Can you work these out from the model? Positions are in its coordinate system, mm. A direction names the side the tool comes from. Round coordinates to 2 decimals unless told otherwise and drop trailing zeros. Order: outer loops, then holes, each group sorted by start corner. A loop starts at its lowest first (then second) coordinate and runs counter-clockwise, first axis right, second up. Notation, with made-up numbers: M 6.25,41.25 L 27.25,41.25 A6 cw 27.25,48.25 Z; hole C -4,78.5 d5. An arc over 180 degrees is marked long. One line per question, with ' | ' between items.
```python
from build123d import *

# Parameters (mm, degrees)
BOSS_EXTRUDE1_DEPTH = 50
SKETCH2_R           = 52
BOSS_EXTRUDE2_DEPTH = 67
SKETCH3_R           = 43
BOSS_EXTRUDE3_DEPTH = 3
CUT_EXTRUDE1_REACH  = 322
SKETCH4_R           = 24
SKETCH5_R           = 33
CUT_EXTRUDE2_DEPTH  = 4
BOSS_EXTRUDE4_DEPTH = 248
SKETCH7_R           = 3
CUT_EXTRUDE3_DEPTH  = 248
BOSS_EXTRUDE5_DEPTH = 20
SKETCH9_R           = 50
BOSS_EXTRUDE6_DEPTH = 20
CUT_EXTRUDE4_REACH  = 22
FILLET1_R           = 25
CUT_EXTRUDE5_DEPTH  = 34
SKETCH12_W          = 78
SKETCH12_H          = 64
CUT_EXTRUDE6_DEPTH  = 240
SKETCH13_W          = 12
SKETCH13_H          = 110
CUT_EXTRUDE7_DEPTH  = 240


with BuildPart() as part:
    # Sketch1 → Boss-Extrude1 (new body, symmetric)
    with BuildSketch(Plane(origin=(0, 0, 0), x_dir=(0, 0, -1), z_dir=(1, 0, 0))):
        with BuildLine():
            Line((-226, 0), (54, 0))
            Line((54, 0), (54, 20))
            Line((54, 20), (52, 20))
            Line((52, 20), (52, 80))
            Line((52, 80), (20, 80))
            Line((20, 80), (20, 74))
            Line((20, 74), (-20, 74))
            Line((-20, 74), (-20, 80))
            Line((-20, 80), (-58, 80))
            Line((-58, 80), (-58, 250))
            Line((-58, 250), (0, 250))
            Line((0, 250), (0, 317))
            Line((0, 317), (-58, 317))
            ThreePointArc((-58, 317), (-114.640297133, 296.941952651), (-146.034066228, 245.708372014))
            Line((-146.034066228, 245.708372014), (-194, 20))
            Line((-194, 20), (-226, 20))
            Line((-226, 20), (-226, 0))
        make_face()
    extrude(amount=BOSS_EXTRUDE1_DEPTH, both=True)

    # Sketch2 → Boss-Extrude2 (add)
    with BuildSketch(Plane(origin=(0, 317, 0), x_dir=(1, 0, 0), z_dir=(0, 1, 0))):
        Circle(SKETCH2_R)
    extrude(amount=-BOSS_EXTRUDE2_DEPTH)

    # Sketch3 → Boss-Extrude3 (add)
    with BuildSketch(Plane(origin=(0, 317, 0), x_dir=(1, 0, 0), z_dir=(0, 1, 0))):
        Circle(SKETCH3_R)
    extrude(amount=BOSS_EXTRUDE3_DEPTH)

    # Sketch4 → Cut-Extrude1 (cut, up to next)
    with BuildSketch(Plane(origin=(0, 320, 0), x_dir=(1, 0, 0), z_dir=(0, 1, 0)), mode=Mode.PRIVATE) as cut_extrude1_sk1:
        Circle(SKETCH4_R)
    cut_extrude1_tool1 = extrude(cut_extrude1_sk1.sketch, amount=-CUT_EXTRUDE1_REACH, mode=Mode.PRIVATE) & part.part
    add(cut_extrude1_tool1.solids().sort_by_distance((0, 320, 0))[0], mode=Mode.SUBTRACT)

    # Sketch5 → Cut-Extrude2 (cut)
    with BuildSketch(Plane.XZ.offset(-250)):
        Circle(SKETCH5_R)
    extrude(amount=-CUT_EXTRUDE2_DEPTH, mode=Mode.SUBTRACT)

    # Sketch6 → Boss-Extrude4 (add, symmetric)
    with BuildSketch(Plane(origin=(0, 0, 0), x_dir=(0, 0, -1), z_dir=(1, 0, 0))):
        Polygon((-58, 80), (-58, 0), (54, 0), (54, 20), (52, 20), (52, 80), (20, 80), (20, 74), (-20, 74), (-20, 80), align=None)
    extrude(amount=BOSS_EXTRUDE4_DEPTH, both=True)

    # Sketch7 → Cut-Extrude3 (cut, symmetric)
    with BuildSketch(Plane(origin=(0, 0, 0), x_dir=(0, 0, -1), z_dir=(1, 0, 0))):
        with Locations((-55, 80)):
            Circle(SKETCH7_R)
    extrude(amount=CUT_EXTRUDE3_DEPTH, both=True, mode=Mode.SUBTRACT)

    # Sketch8 → Boss-Extrude5 (add)
    with BuildSketch(Plane.XZ):
        with BuildLine():
            Line((-272, 12.5), (-303.006817759, 12.5))
            ThreePointArc((-303.006817759, 12.5), (-192, 2), (-303.006817759, -8.5))
            Line((-303.006817759, -8.5), (-272, -8.5))
            ThreePointArc((-272, -8.5), (-261.5, 2), (-272, 12.5))
        make_face()
        with BuildLine():
            Line((272, -8.5), (303.006817759, -8.5))
            ThreePointArc((303.006817759, -8.5), (192, 2), (303.006817759, 12.5))
            Line((303.006817759, 12.5), (272, 12.5))
            ThreePointArc((272, 12.5), (261.5, 2), (272, -8.5))
        make_face()
    extrude(amount=-BOSS_EXTRUDE5_DEPTH)

    # Sketch9 → Boss-Extrude6 (add)
    with BuildSketch(Plane(origin=(0, 20, 0), x_dir=(1, 0, 0), z_dir=(0, 1, 0))):
        with Locations((0, -226)):
            Circle(SKETCH9_R)
    extrude(amount=-BOSS_EXTRUDE6_DEPTH)

    # Sketch10 → Cut-Extrude4 (cut, up to next)
    with BuildSketch(Plane(origin=(0, 20, 0), x_dir=(1, 0, 0), z_dir=(0, 1, 0)), mode=Mode.PRIVATE) as cut_extrude4_sk1:
        with BuildLine():
            ThreePointArc((10.5, -226), (0, -215.5), (-10.5, -226))
            Line((-10.5, -226), (-10.5, -291))
            ThreePointArc((-10.5, -291), (0, -301.5), (10.5, -291))
            Line((10.5, -291), (10.5, -226))
        make_face()
    cut_extrude4_tool1 = extrude(cut_extrude4_sk1.sketch, amount=-CUT_EXTRUDE4_REACH, mode=Mode.PRIVATE) & part.part
    add(cut_extrude4_tool1.solids().sort_by_distance((0, 20, 258.5))[0], mode=Mode.SUBTRACT)

    # Fillet1
    fillet1_edges = [part.edges().sort_by_distance(p)[0] for p in [
        (0, 250, 58),
    ]]
    fillet(fillet1_edges, radius=FILLET1_R)

    # Sketch11 → Cut-Extrude5 (cut, symmetric)
    with BuildSketch(Plane(origin=(0, 0, 0), x_dir=(0, 0, -1), z_dir=(1, 0, 0))):
        with BuildLine():
            Line((-130.383565565, 242.382439212), (-181.892953201, 0))
            Line((-181.892953201, 0), (0, 0))
            Line((0, 0), (0, 64))
            Line((0, 64), (-74, 64))
            Line((-74, 64), (-74, 225))
            ThreePointArc((-74, 225), (-61.991378029, 253.991378029), (-33, 266))
            Line((-33, 266), (-33, 301))
            Line((-33, 301), (-58, 301))
            ThreePointArc((-58, 301), (-104.570910976, 284.507827735), (-130.383565565, 242.382439212))
        make_face()
    extrude(amount=CUT_EXTRUDE5_DEPTH, both=True, mode=Mode.SUBTRACT)

    # Sketch12 → Cut-Extrude6 (cut, symmetric)
    with BuildSketch(Plane(origin=(0, 0, 0), x_dir=(0, 0, -1), z_dir=(1, 0, 0))):
        with Locations((-3, 32)):
            Rectangle(SKETCH12_W, SKETCH12_H)
    extrude(amount=CUT_EXTRUDE6_DEPTH, both=True, mode=Mode.SUBTRACT)

    # Sketch13 → Cut-Extrude7 (cut, symmetric)
    with BuildSketch(Plane(origin=(0, 0, 58), x_dir=(-1, 0, 0), z_dir=(0, 0, -1))):
        with Locations((14, 170)):
            Rectangle(SKETCH13_W, SKETCH13_H)
        with Locations((-14, 170)):
            Rectangle(SKETCH13_W, SKETCH13_H)
    extrude(amount=CUT_EXTRUDE7_DEPTH, both=True, mode=Mode.SUBTRACT)


solid = part.part
```
(1) If we section it at C-C on y = 199: Please give me the cut outline in (x, z), plus the area to 3 significant figures.
Final values:
outline: M -50,58 L -20,58 L -20,74 L -34,74 L -34,139.6 L -20,139.6 L -20,155.96 L -50,155.96 Z; M -8,58 L 8,58 L 8,74 L -8,74 Z; M -8,139.6 L 8,139.6 L 8,155.96 L -8,155.96 Z; M 20,58 L 50,58 L 50,155.96 L 20,155.96 L 20,139.6 L 34,139.6 L 34,74 L 20,74 Z | area: 4,560 mm^2
(2) Thinking about a two-plate mould opening in Y: for faces 5 (the flat face through (14, 225, 142)), 6 (the flat face through (8, 169, 66)), 7 (the flat face through (-14, 115, 166)), 8 (the flat face through (-20, 169, 154)), which applies, released by +Y, released by -Y, zero draft, split by the parting line, or undercut?
Final values:
face 5: released by -Y | face 6: undercut | face 7: released by +Y | face 8: zero draft
(3) If we section it at B-B on z = 0: Please give me the cut outline in (x, y), plus the area to 3 significant figures.
Final values:
outline: M -261.69,0 L -240,0 L -240,64 L 240,64 L 240,0 L 261.69,0 L 261.69,20 L 248,20 L 248,74 L -248,74 L -248,20 L -261.69,20 Z; M -52,250 L -33,250 L -33,254 L -24,254 L -24,320 L -43,320 L -43,317 L -52,317 Z; M 24,254 L 33,254 L 33,250 L 52,250 L 52,317 L 43,317 L 43,320 L 24,320 Z | area: 10,300 mm^2
(4) On a 3-axis mill with a long thin cutter (end or side, diameter ignored), from which of +Z, -Z, +X, -X, +Y, -Y can I reach the whole of each face in a straight line? I mean faces 1 (the flat face through (-14, 115, 66)), 2 (the cylindrical face through (0.48, 253.67, 62.31)), 3 (the cylindrical face through (-5.598, 318.479, -42.634)), 4 (the flat face through (-14, 225, 142)). Say none if no direction works.
Final values:
face 1: +Z, -Z | face 2: none | face 3: +Y | face 4: +Z, -Z, -Y
(5) Will these pins go through, and if not, where does the flat tip stop? pin 1 Ø22 at (x, y) = (-282, 12) entering from -Z; pin 2 Ø9.5 at (x, z) = (-15, 69.5) entering from +Y; pin 3 Ø12 at (y, z) = (45, 75) entering from +X.
Final values:
pin 1: z = -49.06 | pin 2: y = 316.75 | pin 3: x = 50
(6) If we section it at D-D on x = -227.5: Please give me the cut outline in (y, z), plus the area to 3 significant figures.
Final values:
outline: M 0,-54 L 20,-54 L 20,-52 L 80,-52 L 80,-20 L 74,-20 L 74,20 L 80,20 L 80,52 A3 cw 80,58 L 0,58 L 0,42 L 64,42 L 64,-36 L 0,-36 Z | area: 3,590 mm^2
(7) If we section it at A-A on z = 246: Please give me the cut outline in (x, y).
Final values:
outline: M -45.83,0 L -10.5,0 L -10.5,20 L -45.83,20 Z; M 10.5,0 L 45.83,0 L 45.83,20 L 10.5,20 Z
(8) Please list where these lines run through material, in increasing order: probe 1 along Z at (x, y) = (-69, 59); probe 2 along X at (y, z) = (14, 112); probe 3 along X at (y, z) = (283, 0). Write a range as [from, to].
Final values:
probe 1: [-52, -36], [42, 58] | probe 2: [-50, -34], [34, 50] | probe 3: [-52, -24], [24, 52]
